Design review of the part shown in the three views and the two pictorial views. Dimensions are in mm from the part's minimum x, y and z. Give positions to 0.01 mm unless a question says otherwise; leave off trailing zeros. Loops run counter-clockwise (first coordinate to the right, second up) from the corner with the lowest first, then second, coordinate; pieces in that order, holes last. Notation, with made-up numbers: (25, 44) - (78, 44) arc R34 cw to (78, 80) - close; hole circle Ø10 at (4.5, -15.75). An arc over 180 degrees is marked (long way). Use CSV: the item, a comma, the result in double quotes. Start each with the question number.
1. Take a section at C-C on y = 0.25. Give the boundary of the cut face in (x, z).
2. Take a section at B-B on z = 30. Give the boundary of the cut face in (x, y).
3. Take a section at D-D on x = 7.25. Give the boundary of the cut face in (y, z) (1 decimal), plus the area to 3 significant figures.
4. For pin 1 (0.5 mm diameter, centred on y = 0.5, z = 47.5, fed in from +X); pin 2 (3 mm diameter, centred on x = 7.25, z = 5.75, fed in from +Y), all flat-tipped, find the tip position at first contact; note any pin that passes through.
5. Wall thickness on line 1 (X direction, y = 0.8, z = 32); line 2 (X direction, y = 0.85, z = 6) (1 decimal); line 3 (X direction, y = 0.7, z = 5.75): over which ranges is each line inside the solid? List them lowest first.
6. Take a section at A-A on x = 67. Give the boundary of the cut face in (y, z).
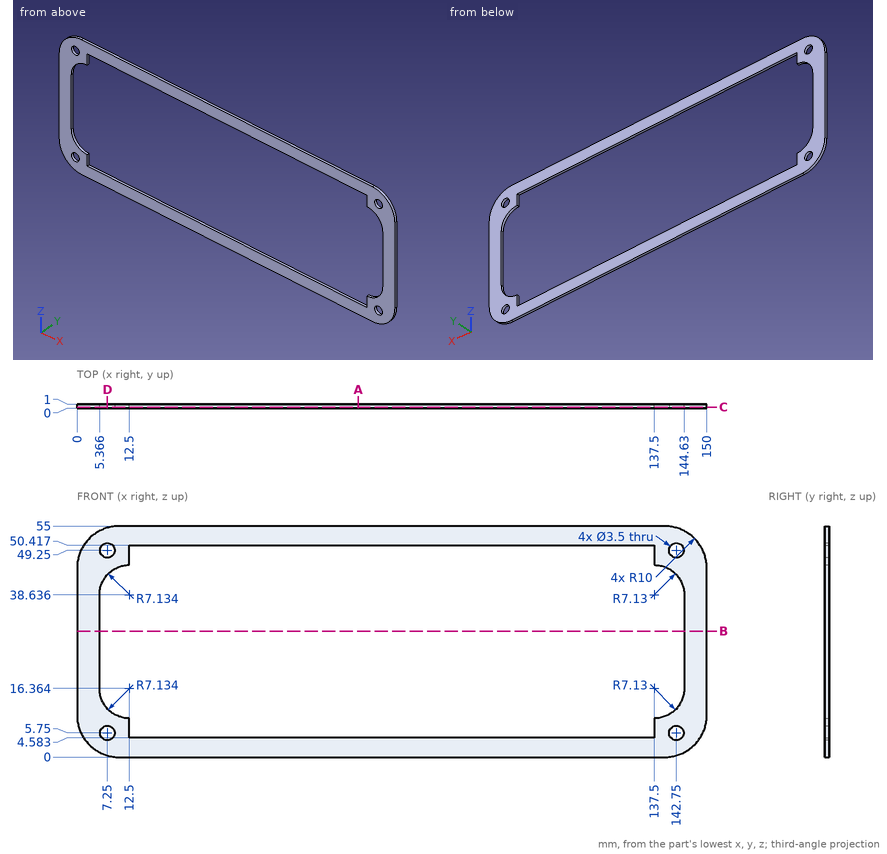
Check result:
1,outline,"(0, 10) arc R10 ccw to (10, 0) - (140, 0) arc R10 ccw to (150, 10) - (150, 45) arc R10 ccw to (140, 55) - (10, 55) arc R10 ccw to (0, 45) - close; hole (5.37, 16.36) arc R7.13 ccw to (12.5, 9.23) - (12.5, 4.58) - (137.5, 4.58) - (137.5, 9.23) arc R7.13 ccw to (144.63, 16.36) - (144.63, 38.64) arc R7.13 ccw to (137.5, 45.77) - (137.5, 50.42) - (12.5, 50.42) - (12.5, 45.77) arc R7.13 ccw to (5.37, 38.64) - close; hole circle Ø3.5 at (7.25, 5.75); hole circle Ø3.5 at (7.25, 49.25); hole circle Ø3.5 at (142.75, 5.75); hole circle Ø3.5 at (142.75, 49.25)"
2,outline,"(0, 0) - (5.37, 0) - (5.37, 1) - (0, 1) - close; (144.63, 0) - (150, 0) - (150, 1) - (144.63, 1) - close"
3,outline,"(0, 0.4) - (1, 0.4) - (1, 4) - (0, 4) - close; (0, 7.5) - (1, 7.5) - (1, 11.5) - (0, 11.5) - close; (0, 43.5) - (1, 43.5) - (1, 47.5) - (0, 47.5) - close; (0, 51) - (1, 51) - (1, 54.6) - (0, 54.6) - close"
3,area,"15.3 mm²"
4,pin 1,"stops at x = 149.74"
4,pin 2,"passes through"
5,line 1,"x = 0 to 5.37, 144.63 to 150"
5,line 2,"x = 0.8 to 5.5, 9 to 12.5, 137.5 to 141, 144.5 to 149.2"
5,line 3,"x = 0.95 to 5.5, 9 to 12.5, 137.5 to 141, 144.5 to 149.05"
6,outline,"(0, 0) - (1, 0) - (1, 4.58) - (0, 4.58) - close; (0, 50.42) - (1, 50.42) - (1, 55) - (0, 55) - close"
